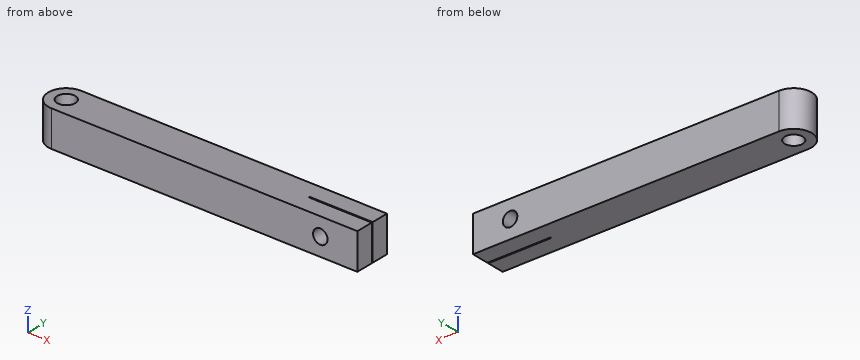
```python
from build123d import *

# Parameters (mm, degrees)
SKETCH1_R              = 3.175
BOSS_EXTRUDE1_DEPTH    = 12.7
F_10_CLEARANCE_HOLE2_D = 5.1054


with BuildPart() as part:
    # Sketch1 → Boss-Extrude1 (new body)
    with BuildSketch(Plane.XY):
        with BuildLine():
            Line((85.725, 0.1905), (85.725, -0.1905))
            Line((85.725, -0.1905), (107.95, -0.1905))
            Line((107.95, -0.1905), (107.95, -6.35))
            Line((107.95, -6.35), (7.14e-07, -6.35))
            ThreePointArc((7.14e-07, -6.35), (-6.35, -3.57e-07), (0, 6.35))
            Line((0, 6.35), (107.95, 6.35))
            Line((107.95, 6.35), (107.95, 0.1905))
            Line((107.95, 0.1905), (85.725, 0.1905))
        make_face()
        Circle(SKETCH1_R, mode=Mode.SUBTRACT)
    extrude(amount=BOSS_EXTRUDE1_DEPTH)

    # #10 Clearance Hole2 (through all)
    with Locations(Plane(origin=(0, 6.35, 0), x_dir=(1, 0, 0), z_dir=(0, 1, 0))):
        with Locations((94.869, -6.35)):
            Hole(F_10_CLEARANCE_HOLE2_D / 2)


solid = part.part
```
For this review, take the finished solid that the model builds, in its own axes (mm). Coordinates: 2 decimals unless noted, no trailing zeros. Write each loop counter-clockwise with the first axis right and the second up, starting at its lowest first coordinate (ties: lowest second). Pieces come first, ordered by that corner, then holes. Notation, with made-up numbers: (38.25, 5) - (47.25, 5) arc R10 ccw to (47.25, 21) - close; hole circle Ø5 at (62.5, 30). An arc over 180 degrees is marked (long way). Answer in a Markdown table with one row per item. Add a question column.
Q1. We need section C-C, the plane y = 2. State the section outline as (x, z) points, and give its area (3 significant figures).
Q2. We need section A-A, the plane z = 6.35. Count the separate pieces of the cut face and the enclosed holes in it, and give its area (3 significant figures).
Q3. We need section B-B, the plane x = 88.5. State the section outline as (y, z) points, and give its area (3 significant figures).
Q4. For probe 1 along Y at (x, z) = (103, 4.25); probe 2 along X at (y, z) = (0.25, 10); probe 3 along X at (y, z) = (4.75, 6), list the stretches that pass through material, from the lowest coordinate up.
Q5. For P1, Ø6.5, axis at x = 96.5, z = 5.5, coming from the +Y side; P2, Ø1.5, axis at y = -3, z = 1.5, coming from the -X side, all flat-tipped, find the tip position at first contact; note any pin that passes through.
Answer list:
| question | item | result |
|---|---|---|
| 1 | outline | (-6.03, 0) - (-2.47, 0) - (-2.47, 12.7) - (-6.03, 12.7) - close; (2.47, 0) - (107.95, 0) - (107.95, 12.7) - (2.47, 12.7) - close; hole circle Ø5.11 at (94.87, 6.35) |
| 1 | area | 1,360 mm2 |
| 2 | separate pieces | 3 |
| 2 | enclosed holes | 1 |
| 2 | area | 1,330 mm2 |
| 3 | outline | (-6.35, 0) - (-0.19, 0) - (-0.19, 12.7) - (-6.35, 12.7) - close; (0.19, 0) - (6.35, 0) - (6.35, 12.7) - (0.19, 12.7) - close |
| 3 | area | 156 mm2 |
| 4 | probe 1 | y = -6.35 to -0.19, 0.19 to 6.35 |
| 4 | probe 2 | x = -6.35 to -3.17, 3.17 to 107.95 |
| 4 | probe 3 | x = -4.21 to 92.34, 97.4 to 107.95 |
| 5 | P1 | stops at y = 6.35 |
| 5 | P2 | stops at x = -5.94 |
